Verification items for the finished model (mm, model axes). Face numbers are marked on the shaded views. A direction names the side the tool comes from. Round coordinates to 2 decimals unless told otherwise and drop trailing zeros. Write each loop counter-clockwise with the first axis right and the second up, starting at its lowest first coordinate (ties: lowest second). Pieces come first, ordered by that corner, then holes. Notation, with made-up numbers: (71, 57) - (124, 57) arc R21 cw to (124, 94) - close; hole circle Ø2 at (43.25, 35). An arc over 180 degrees is marked (long way). Write each question's results on one line, items separated by ' | '.
```python
from build123d import *

# Parameters (mm, degrees)
F1_DEPTH = 19.05
F2_D     = 139.999974
F2_DEPTH = 50.8
F2_TIP   = 42.0602355207


with BuildPart() as f1:
    # F0 (on Right) → F1 (new body)
    with BuildSketch(Plane.YZ):
        Polygon((110.4406434166, 38.438666836), (110.4406434166, 96.266), (-84.3773565834, 96.266), (-84.3773565834, 38.438666836), (-65.3273565834, 38.438666836), (-65.3273565834, -19.388666836), (-84.3773565834, -19.388666836), (-84.3773565834, -77.216), (-19.4380147834, -77.216), (-19.4380147834, -96.266), (45.5013016166, -96.266), (45.5013016166, -77.216), (110.4406434166, -77.216), (110.4406434166, -19.388666836), (91.3906434166, -19.388666836), (91.3906434166, 38.438666836), align=None)
    extrude(amount=F1_DEPTH)

    # F2
    with Locations(Plane(origin=(0, 0, 0), x_dir=(0, 1, 0), z_dir=(-1, 0, 0))):
        with Locations((13.0316434166, -9.525)):
            Hole(F2_D / 2, depth=F2_DEPTH)
            with Locations((0, 0, -(F2_DEPTH + F2_TIP / 2))):  # 118° drill point
                Cone(0, F2_D / 2, F2_TIP, mode=Mode.SUBTRACT)


solid = f1.part
```
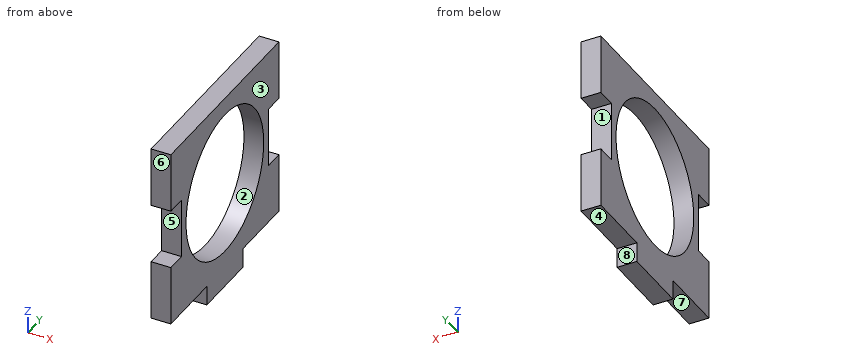
(1) Go/stop test with flat-tipped pins: pin 1 Ø9.5 at (x, z) = (12, -3.5) entering from +Y; pin 2 Ø1.5 at (y, z) = (23.5, -59.5) entering from +X; pin 3 Ø5.5 at (x, z) = (7, -88.5) entering from -Y; pin 4 Ø5.5 at (x, z) = (9, -89) entering from +Y. Record where each tip stops, or that it passes through.
Answer:
pin 1: y = 91.39 | pin 2: x = 19.05 | pin 3: y = -19.44 | pin 4: y = 45.5
(2) Section check C-C (x = 7). Record the cut outline in (y, z) (3 decimals).
Answer:
outline: (-84.377, -77.216) - (-19.438, -77.216) - (-19.438, -96.266) - (45.501, -96.266) - (45.501, -77.216) - (110.441, -77.216) - (110.441, -19.389) - (91.391, -19.389) - (91.391, 38.439) - (110.441, 38.439) - (110.441, 96.266) - (-84.377, 96.266) - (-84.377, 38.439) - (-65.327, 38.439) - (-65.327, -19.389) - (-84.377, -19.389) - close; hole circle Ø140 at (13.032, 9.525)
(3) Thickness scan on L1, parallel to Z at x = 12.5, y = 86.5; L2, parallel to Y at x = 14.5, z = -40.5; L3, parallel to Y at x = 15.75, z = -27. Record the ranges inside material, lowest first.
Answer:
L1: -77.22 to 96.27 | L2: -84.38 to -35.93, 62 to 110.44 | L3: -84.38 to -46.68, 72.75 to 110.44
(4) Section check A-A (y = 98). Record the cut outline in (x, z).
Answer:
outline: (0, -77.22) - (19.05, -77.22) - (19.05, -19.39) - (0, -19.39) - close; (0, 38.44) - (19.05, 38.44) - (19.05, 96.27) - (0, 96.27) - close
(5) Mould release check, pull along Z, two halves, no side actions. Record for the marked faces 1, 2, 3 and 4: released by +Z, released by -Z, zero draft, split by the parting line, or undercut.
Answer:
face 1: undercut | face 2: undercut | face 3: zero draft | face 4: released by -Z
(6) Section check B-B (z = 69.5). Record the cut outline in (x, y), plus the area to 3 significant figures.
Answer:
outline: (0, -84.38) - (19.05, -84.38) - (19.05, -23.07) - (0, -23.07) - close; (0, 49.13) - (19.05, 49.13) - (19.05, 110.44) - (0, 110.44) - close | area: 2,340 mm2
(7) Set-up check for the marked faces 5, 6, 7 and 8: record each of +Z, -Z, +X, -X, +Y, -Y from which the full face is reachable in a straight line by a thin tool's end or side.
Answer:
face 5: +X, -X, -Y | face 6: +Z, -Z, +X, -X, -Y | face 7: -Z, +X, -X, -Y | face 8: -Z, +X, -X, +Y
